Autodesk Inventor part; units mm, degrees
ref_plane "YZ Plane" through (0, 0, 0) normal (1, 0, 0) x (0, 1, 0)
ref_plane "XZ Plane" through (0, 0, 0) normal (0, 1, 0) x (-1, 0, 0)
ref_plane "XY Plane" through (0, 0, 0) normal (0, 0, 1) x (1, 0, 0)
sketch "Sketch1" plane through (0, 0, 0) normal (1, 0, 0) x (0, 1, 0)
  line L0 (0, 10) -> (4, 10)
  line L1 (4, 10) -> (4, 0)
  line L2 (4, 0) -> (5, 0)
  line L3 (5, 0) -> (5, -40)
  line L4 (5, -40) -> (4, -40)
  line L5 (4, -40) -> (4, -50)
  line L6 (4, -50) -> (0, -50)
  line L7 (0, -50) -> (0, 10)
  point P0 (0, 0)
  dimension "d0" = 4
  dimension "d1" = 10
  dimension "d2" = 10
  dimension "d3" = 5
  dimension "d4" = 0
  dimension "d5" = 0
  dimension "d6" = 40
revolve "Revolution1" add sketch "Sketch1" angle 360 about axis through (0, 0, -50) along (0, 0, 1)
properties part number "eixo"
Check sheet for the modelled part. Datum: model origin and axes. Units: mm. A direction names the side the tool comes from. Give positions to 0.01 mm unless a question says otherwise; leave off trailing zeros. Write each loop counter-clockwise with the first axis right and the second up, starting at its lowest first coordinate (ties: lowest second). Pieces come first, ordered by that corner, then holes. Notation, with made-up numbers: (26, 30.25) -> (50, 30.25) arc R26 ccw to (50, 65.25) -> close; hole circle Ø6 at (-22.5, 27.5). An arc over 180 degrees is marked (long way). Use one line per item in the form item = value. Start each with the question number.
1. Access from +Z, -Z, +X, -X, +Y, -Y to the whole of each face (thin tool, end or side, straight path). Record for faces 1 (the flat face through (0, 0, -50)), 2 (the cylindrical face through (-3.905, -0.867, 4.93)), 3 (the cylindrical face through (-3.905, -0.867, -45.07)).
2. Go/stop test with a flat-tipped pin: P1, Ø2, axis at x = -0.5, z = -18.5, coming from the +Y side. Record where the tip stops, or that it passes through.
3. Section check D-D (z = -5). Record the cut outline in (x, y), and give its area (3 significant figures).
4. Thickness scan on line 1 along X through (y, z) = (0.25, -42); line 2 along Z through (x, y) = (-1.5, -4.5); line 3 along Y through (x, z) = (-0.25, -17.5). Record the ranges inside material, lowest first. Write a range as from..to.
5. Section check C-C (z = -44). Record the cut outline in (x, y).
6. Section check A-A (x = 0). Record the cut outline in (y, z).
Conclusion:
q1.face_1 = -Z, +X, -X, +Y, -Y
q1.face_2 = +Z
q1.face_3 = -Z
q2.P1 = 5
q3.outline = circle Ø10 at (0, 0)
q3.area = 78.5 mm²
q4.line_1 = -3.99..3.99
q4.line_2 = -40..0
q4.line_3 = -4.99..4.99
q5.outline = circle Ø8 at (0, 0)
q6.outline = (-5, -40) -> (-4, -40) -> (-4, -50) -> (4, -50) -> (4, -40) -> (5, -40) -> (5, 0) -> (4, 0) -> (4, 10) -> (-4, 10) -> (-4, 0) -> (-5, 0) -> close
